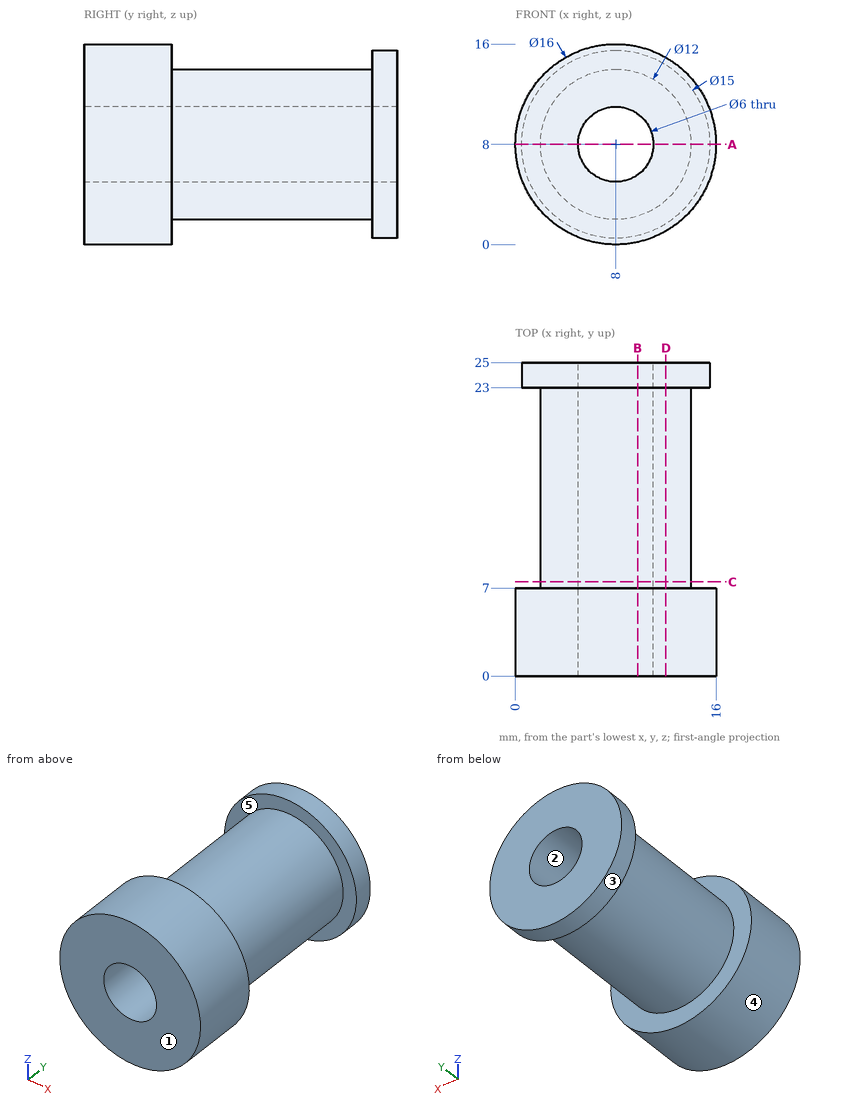
Here's the drawing with two shaded views (mm, measured from the low corner). I have some questions. A direction names the side the tool comes from. Round coordinates to 2 decimals unless told otherwise and drop trailing zeros. Order: outer loops, then holes, each group sorted by start corner. A loop starts at its lowest first (then second) coordinate and runs counter-clockwise, first axis right, second up. Notation, with made-up numbers: M 37,4.25 L 81,4.25 A19 cw 81,22.25 Z; hole C 87.25,88 d8. An arc over 180 degrees is marked long. Answer in a Markdown table with one row per item.
Item 1: Thinking about a two-plate mould opening in X: for the marked faces 1, 2 and 3, which applies, +X half, -X half, draft (parallel to the pull), parting line (faces both ways), or undercut?
A:
| item | result |
|---|---|
| face 1 | draft |
| face 2 | undercut |
| face 3 | parting line |
Item 2: Imagine slicing it at C-C, the plane y = 7.5. Write out the boundary of the cut face in (x, z), and give its area (3 significant figures).
A:
| item | result |
|---|---|
| outline | C 8,8 d12; hole C 8,8 d6 |
| area | 84.8 mm2 |
Item 3: I'm going to push flat-ended pins straight in: pin 1 (5.5 mm diameter, centred on x = 8, z = 8, fed in from +Y); pin 2 (3 mm diameter, centred on y = 14, z = 12.5, fed in from -X); pin 3 (2 mm diameter, centred on y = 20, z = 8, fed in from -X); pin 4 (1.5 mm diameter, centred on y = 10.5, z = 11, fed in from +X). Where does each tip first touch, or does it pass through?
A:
| item | result |
|---|---|
| pin 1 | passes through |
| pin 2 | stops at x = 2.8 |
| pin 3 | stops at x = 2 |
| pin 4 | stops at x = 13.56 |
Item 4: Imagine slicing it at A-A, the plane z = 8. Write out the boundary of the cut face in (x, y).
A:
| item | result |
|---|---|
| outline | M 0,0 L 5,0 L 5,25 L 0.5,25 L 0.5,23 L 2,23 L 2,7 L 0,7 Z; M 11,0 L 16,0 L 16,7 L 14,7 L 14,23 L 15.5,23 L 15.5,25 L 11,25 Z |
Item 5: Imagine slicing it at B-B, the plane x = 9.75. Write out the boundary of the cut face in (y, z), and give its area (3 significant figures).
A:
| item | result |
|---|---|
| outline | M 0,0.19 L 7,0.19 L 7,2.26 L 23,2.26 L 23,0.71 L 25,0.71 L 25,5.56 L 0,5.56 Z; M 0,10.44 L 25,10.44 L 25,15.29 L 23,15.29 L 23,13.74 L 7,13.74 L 7,15.81 L 0,15.81 Z |
| area | 200 mm2 |
Item 6: If I drill on L1, parallel to Y at x = 7.5, z = 14.25; L2, parallel to X at y = 19, z = 8; L3, parallel to X at y = 6.25, z = 5.25, over which ranges is the centre line in solid material (lowest first)? Write a range as from..to.
A:
| item | result |
|---|---|
| L1 | y = 0..7, 23..25 |
| L2 | x = 2..5, 11..14 |
| L3 | x = 0.49..6.8, 9.2..15.51 |
Item 7: For the marked faces 4 and 5, which set-ups out of +Z, -Z, +X, -X, +Y, -Y let a thin tool reach every point of the face, with its end or its side?
A:
| item | result |
|---|---|
| face 4 | +Y, -Y |
| face 5 | none |
Item 8: Imagine slicing it at D-D, the plane x = 12. Write out the boundary of the cut face in (y, z).
A:
| item | result |
|---|---|
| outline | M 0,1.07 L 7,1.07 L 7,3.53 L 23,3.53 L 23,1.66 L 25,1.66 L 25,14.34 L 23,14.34 L 23,12.47 L 7,12.47 L 7,14.93 L 0,14.93 Z |
